Design review of the part shown in the three views and the two pictorial views. Dimensions are in mm from the part's minimum x, y and z. Round coordinates to 2 decimals unless told otherwise and drop trailing zeros. Loops run counter-clockwise (first coordinate to the right, second up) from the corner with the lowest first, then second, coordinate; pieces in that order, holes last. Notation, with made-up numbers: M -26,64 L -12,64 A18 cw -12,80 Z; hole C -38.75,89.5 d4. An arc over 180 degrees is marked long. Return JSON: item names as keys, results as strings. Group by question number.
Q1. Consider section A-A (x = 13.25). State the section outline as (y, z) points.
Q2. Draft analysis for pull direction X (two halves, no side actions). For the marked faces 1 and 2, state which applies: pulls with the +X half, pulls with the -X half, needs draft (parallel to the pull), parting line crosses it, or undercut.
Q3. Consider section C-C (z = 1.75). State the section outline as (x, y) points, and give its area (3 significant figures).
Q4. To check wall thickness, follow line 1 along Y through (x, z) = (13.25, 1.5); line 2 along X through (y, z) = (7.5, 3); line 3 along Y through (x, z) = (11.5, 4.5). State the ranges of each line that lie inside material, in increasing order.
Q5. Consider section B-B (y = 4.8). State the section outline as (x, z) points, and give its area (3 significant figures).
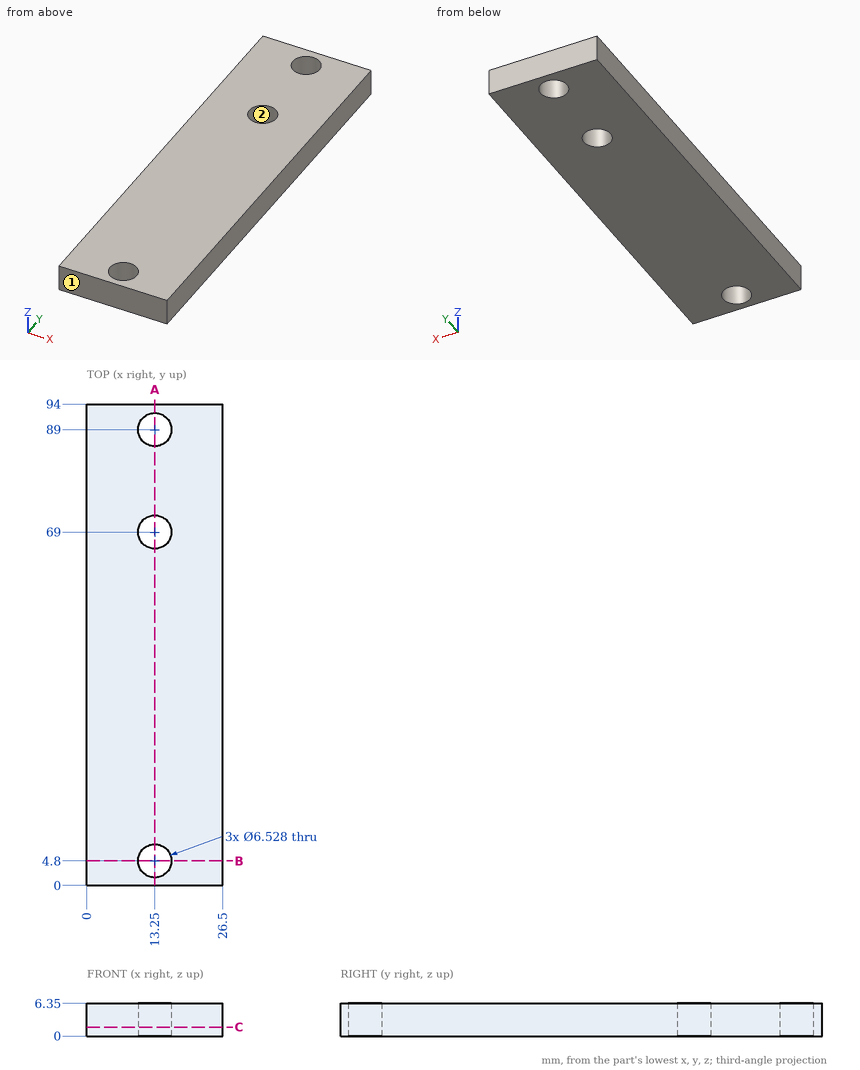
Values:
{
 "1": {"outline": "M 0,0 L 1.54,0 L 1.54,6.35 L 0,6.35 Z; M 8.06,0 L 65.74,0 L 65.74,6.35 L 8.06,6.35 Z; M 72.26,0 L 85.74,0 L 85.74,6.35 L 72.26,6.35 Z; M 92.26,0 L 94,0 L 94,6.35 L 92.26,6.35 Z"},
 "2": {"face 1": "needs draft", "face 2": "undercut"},
 "3": {"outline": "M 0,0 L 26.5,0 L 26.5,94 L 0,94 Z; hole C 13.25,4.8 d6.53; hole C 13.25,69 d6.53; hole C 13.25,89 d6.53", "area": "2,390 mm2"},
 "4": {"line 1": "y = 0 to 1.54, 8.06 to 65.74, 72.26 to 85.74, 92.26 to 94", "line 2": "x = 0 to 11.42, 15.08 to 26.5", "line 3": "y = 0 to 2.04, 7.56 to 66.24, 71.76 to 86.24, 91.76 to 94"},
 "5": {"outline": "M 0,0 L 9.99,0 L 9.99,6.35 L 0,6.35 Z; M 16.51,0 L 26.5,0 L 26.5,6.35 L 16.51,6.35 Z", "area": "127 mm2"}
}
